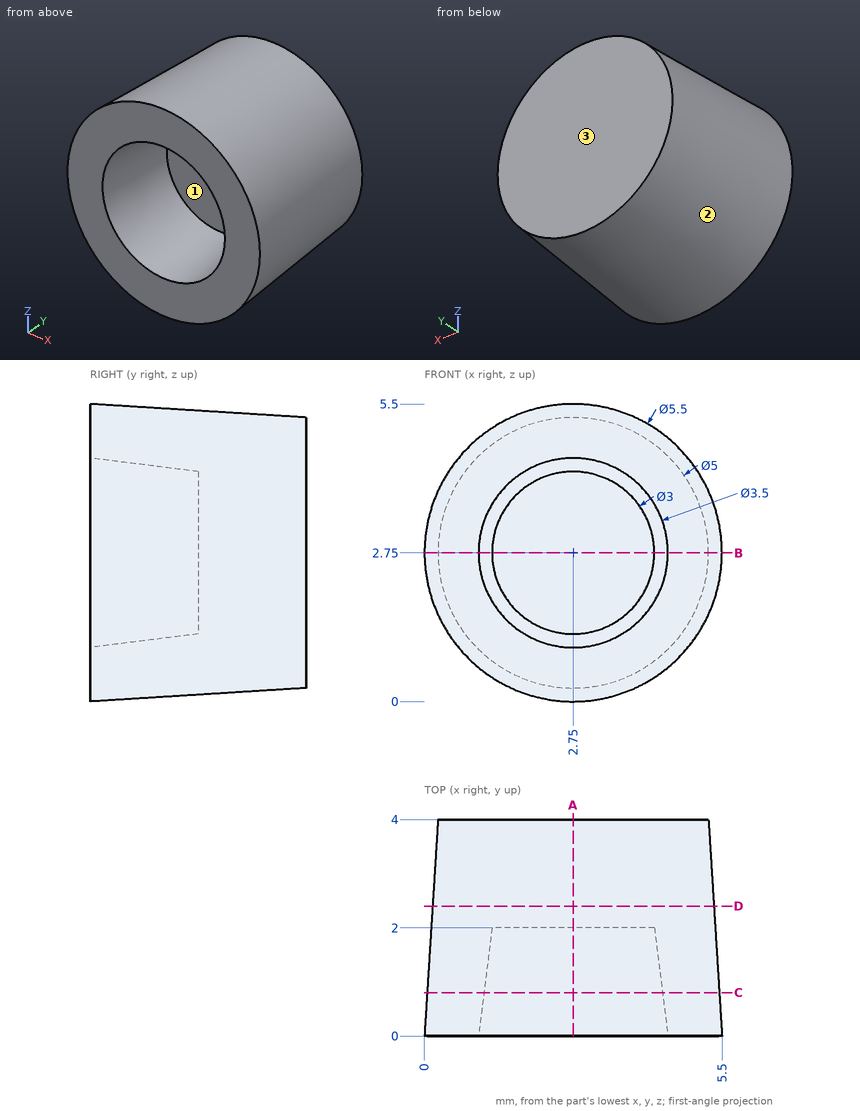
Study the drawing (mm; zero at the part's minimum x, y, z) and answer. Give positions to 0.01 mm unless a question says otherwise; leave off trailing zeros. Order: outer loops, then holes, each group sorted by start corner. A loop starts at its lowest first (then second) coordinate and runs counter-clockwise, first axis right, second up.
1) Find section B-B on z = 2.75. Write down the section's boundary in (x, y), then the cut area to 3 significant figures.
Reported:
outline: (0, 0) - (1, 0) - (1.25, 2) - (4.25, 2) - (4.5, 0) - (5.5, 0) - (5.25, 4) - (0.25, 4) - close
area: 14.5 mm2
2) Find section C-C on y = 0.8. Write down the section's boundary in (x, z), then the cut area to 3 significant figures.
Reported:
outline: circle Ø5.4 at (2.75, 2.75); hole circle Ø3.3 at (2.75, 2.75)
area: 14.3 mm2
3) Determine the mould class of the marked faces 1, 2 and 3 for opening direction X: pulls with the +X half, pulls with the -X half, needs draft (parallel to the pull), parting line crosses it, or undercut.
Reported:
face 1: undercut
face 2: parting line crosses it
face 3: needs draft
4) Given P1, Ø1.5, axis at y = 0.5, z = 1, coming from the -X side, flat-ended and moving along its own axis, determine where the tip first touches the part or whether it passes through.
Reported:
P1: stops at x = 0.22
5) Find section D-D on y = 2.4. Write down the section's boundary in (x, z), then the cut area to 3 significant figures.
Reported:
outline: circle Ø5.2 at (2.75, 2.75)
area: 21.2 mm2
6) Consider line 1 along X through (y, z) = (1.7, 3.95); line 2 along X through (y, z) = (1.1, 1.75); line 3 along Z through (x, y) = (3.6, 0.7). Determine where each line is inside the solid, lowest interval first.
Reported:
line 1: x = 0.39 to 1.79, 3.71 to 5.11
line 2: x = 0.26 to 1.49, 4.01 to 5.24
line 3: z = 0.18 to 1.32, 4.18 to 5.32
7) Find section A-A on x = 2.75. Write down the section's boundary in (y, z), then the cut area to 3 significant figures.
Reported:
outline: (0, 0) - (4, 0.25) - (4, 5.25) - (0, 5.5) - (0, 4.5) - (2, 4.25) - (2, 1.25) - (0, 1) - close
area: 14.5 mm2
